from build123d import *

# Parameters (mm, degrees)
F1_DEPTH = 4
F2_DEPTH = 2.5
F4_W     = 1
F4_H     = 1.5
F6_W     = 1
F6_H     = 1.5
F8_W     = 5
F8_H     = 5
F9_DEPTH = 2


with BuildPart() as f1:
    # F0 (on Right) → F1 (new body)
    with BuildSketch(Plane.YZ):
        with BuildLine():
            Line((0, 2), (0, 0))
            Line((0, 0), (1.5, 0))
            Line((1.5, 0), (1.5, 1.5845440408))
            ThreePointArc((1.5, 1.5845440408), (7.8976750419, 4.0885304442), (14.5, 5.9883985969))
            Line((14.5, 5.9883985969), (14.5, 0))
            Line((14.5, 0), (16, 0))
            Line((16, 0), (16, 3))
            Line((16, 3), (16, 6.3291188198))
            ThreePointArc((16, 6.3291188198), (19.2376865014, 6.9540783828), (22.5, 7.4341814697))
            Line((22.5, 7.4341814697), (22.5, 3))
            Line((22.5, 3), (24, 3))
            Line((24, 3), (24, 6))
            Line((24, 6), (24, 7.6053708135))
            ThreePointArc((24, 7.6053708135), (27.2457445405, 7.8702512613), (30.5, 7.9920735832))
            Line((30.5, 7.9920735832), (30.5, 6))
            Line((30.5, 6), (32, 6))
            Line((32, 6), (32, 9))
            ThreePointArc((32, 9), (15.6131705465, 7.2683632159), (0, 2))
        make_face()
        with BuildLine():
            Line((1.5, 1.5845440408), (1.5, 0))
            Line((1.5, 0), (14.5, 0))
            Line((14.5, 0), (14.5, 5.9883985969))
            ThreePointArc((14.5, 5.9883985969), (7.8976750419, 4.0885304442), (1.5, 1.5845440408))
        make_face()
        with BuildLine():
            Line((16, 6.3291188198), (16, 3))
            Line((16, 3), (22.5, 3))
            Line((22.5, 3), (22.5, 7.4341814697))
            ThreePointArc((22.5, 7.4341814697), (19.2376865014, 6.9540783828), (16, 6.3291188198))
        make_face()
        with BuildLine():
            Line((24, 6), (30.5, 6))
            Line((30.5, 6), (30.5, 7.9920735832))
            ThreePointArc((30.5, 7.9920735832), (27.2457445405, 7.8702512613), (24, 7.6053708135))
            Line((24, 7.6053708135), (24, 6))
        make_face()
    extrude(amount=F1_DEPTH)

    # F0 (on Right) → F2 (cut)
    with BuildSketch(Plane.YZ):
        with BuildLine():
            Line((24, 6), (30.5, 6))
            Line((30.5, 6), (30.5, 7.9920735832))
            ThreePointArc((30.5, 7.9920735832), (27.2457445405, 7.8702512613), (24, 7.6053708135))
            Line((24, 7.6053708135), (24, 6))
        make_face()
        with BuildLine():
            Line((16, 6.3291188198), (16, 3))
            Line((16, 3), (22.5, 3))
            Line((22.5, 3), (22.5, 7.4341814697))
            ThreePointArc((22.5, 7.4341814697), (19.2376865014, 6.9540783828), (16, 6.3291188198))
        make_face()
        with BuildLine():
            Line((1.5, 1.5845440408), (1.5, 0))
            Line((1.5, 0), (14.5, 0))
            Line((14.5, 0), (14.5, 5.9883985969))
            ThreePointArc((14.5, 5.9883985969), (7.8976750419, 4.0885304442), (1.5, 1.5845440408))
        make_face()
    extrude(amount=F2_DEPTH, mode=Mode.SUBTRACT)

    # F3: F1 across face


with BuildPart() as f1_1:
    add(f1.part)
    add(f1.part.mirror(Plane(origin=(0, 16.947812772, 5.3752677136), x_dir=(0, 1, 0), z_dir=(-1, 0, 0))))

    # F4 (on face) → F5 (join, up to the next surface of F1)
    with BuildSketch(Plane(origin=(0, 0, 6), x_dir=(1, 0, 0), z_dir=(0, 0, -1))):
        with Locations((0, -24.75)):
            Rectangle(F4_W, F4_H)
    extrude(until=Until.NEXT, dir=(0, 0, 1))

    # F6 (on face) → F7 (join, up to the next surface of F1)
    with BuildSketch(Plane(origin=(0, 0, 3), x_dir=(1, 0, 0), z_dir=(0, 0, -1))):
        with Locations((0, -16.75)):
            Rectangle(F6_W, F6_H)
    extrude(until=Until.NEXT, dir=(0, 0, 1))

    # F8 (on face) → F9 (cut)
    with BuildSketch(Plane(origin=(0, 0, 0), x_dir=(1, 0, 0), z_dir=(0, 0, -1))):
        with Locations((0, -4)):
            Rectangle(F8_W, F8_H)
    extrude(amount=-F9_DEPTH, mode=Mode.SUBTRACT)


solid = f1_1.part
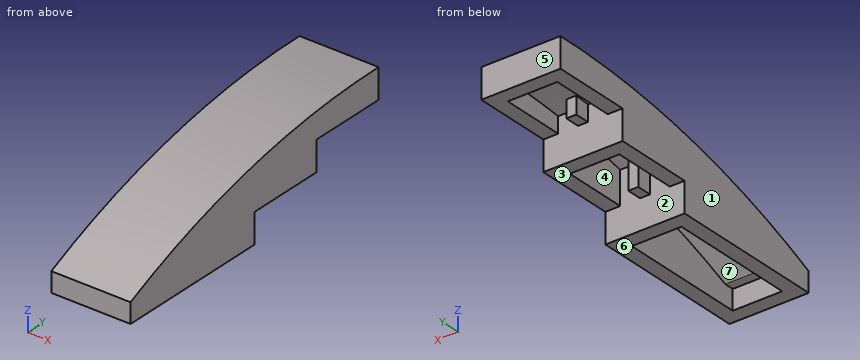
Can you work these out from the model? Positions are in its coordinate system, mm. Face numbers are marked on the shaded views. A direction names the side the tool comes from. Give positions to 0.01 mm unless a question says otherwise; leave off trailing zeros. Order: outer loops, then holes, each group sorted by start corner. A loop starts at its lowest first (then second) coordinate and runs counter-clockwise, first axis right, second up. Notation, with made-up numbers: M 68.5,-2 L 76.5,-2 A12 ccw 76.5,21 Z; hole C 82,13 d11. An arc over 180 degrees is marked long. Use one line per item in the form item = value. Start each with the question number.
Item 1: If we section it at D-D (z = 2.5): Write out the boundary of the cut face in (x, y), then the cut area to 3 significant figures.
Item 2: Will these pins go through, and if not, where does the flat tip stop? pin 1 Ø1 at (x, y) = (-3, 10) entering from +Z; pin 2 Ø1.1 at (x, y) = (0, 24.5) entering from -Z; pin 3 Ø1.4 at (x, z) = (0.5, 4.5) entering from +Y.
Item 3: If we section it at A-A (x = 1): Write out the boundary of the cut face in (y, z).
Item 4: If we section it at B-B (z = 4.5): Write out the boundary of the cut face in (x, y), then the cut area to 3 significant figures.
Item 5: We'd pull the mould along Y, two halves only. Please class the marked faces 4, 5, 6 and 7: +Y half, -Y half, draft (parallel to the pull), parting line (faces both ways), or undercut.
Item 6: If we section it at C-C (y = 13): Write out the boundary of the cut face in (x, z), then the cut area to 3 significant figures.
Item 7: For the marked faces 1, 2 and 3, which set-ups out of +Z, -Z, +X, -X, +Y, -Y let a thin tool reach every point of the face, with its end or its side?
Item 8: If I drill on line 1 along Y through (x, z) = (0, 1.75); line 2 along X through (y, z) = (18.5, 4.5); line 3 along Y through (x, z) = (3.25, 1.75), over which ranges is the centre line in solid material (lowest first)?
Outcome:
q1.outline = M -4,1.1 L 4,1.1 L 4,16 L -4,16 Z; hole M -2.5,3.64 L 2.5,3.64 L 2.5,14.5 L -2.5,14.5 Z
q1.area = 64.9 mm2
q2.pin_1 = 5.96
q2.pin_2 = 3
q2.pin_3 = 24
q3.outline = M 0,0 L 1.5,0 L 1.5,2 L 2.45,2 A74 cw 14.5,5.99 L 14.5,0 L 16,0 L 16,6.33 A74 cw 22.5,7.43 L 22.5,3 L 24,3 L 24,7.61 A74 cw 30.5,7.99 L 30.5,6 L 32,6 L 32,9 A75 ccw 0,2 Z
q4.outline = M -4,6.05 L 4,6.05 L 4,24 L -4,24 Z; hole M -2.5,9.15 L 2.5,9.15 L 2.5,14.5 L -2.5,14.5 Z; hole M -2.5,16 L -0.5,16 L -0.5,17.5 L 0.5,17.5 L 0.5,16 L 2.5,16 L 2.5,22.5 L -2.5,22.5 Z
q4.area = 85.8 mm2
q5.face_4 = undercut
q5.face_5 = +Y half
q5.face_6 = draft
q5.face_7 = undercut
q6.outline = M -4,0 L -2.5,0 L -2.5,5.61 L 2.5,5.61 L 2.5,0 L 4,0 L 4,6.65 L -4,6.65 Z
q6.area = 25.1 mm2
q7.face_1 = +Z, -Z, -X, +Y, -Y
q7.face_2 = -Z
q7.face_3 = -Z, +X, -X, +Y
q8.line_1 = 0 to 1.5, 14.5 to 16
q8.line_2 = -4 to -2.5, 2.5 to 4
q8.line_3 = 0 to 16
